Autodesk Inventor part; units mm, degrees
ref_plane "YZ Plane" through (0, 0, 0) normal (1, 0, 0) x (0, 1, 0)
ref_plane "XZ Plane" through (0, 0, 0) normal (0, 1, 0) x (-1, 0, 0)
ref_plane "XY Plane" through (0, 0, 0) normal (0, 0, 1) x (1, 0, 0)
sketch "Sketch1" plane through (0, 0, 0) normal (0, 0, 1) x (1, 0, 0)
  circle A0 centre (0, 0) radius 30
  dimension "d0" = 60
extrude "Extrusion1" add sketch "Sketch1" along normal mid plane 58.037
sketch "Sketch2" plane through (0, 0, 0) normal (0, 0, 1) x (1, 0, 0)
  circle A0 centre (0, 0) radius 30
  circle A1 centre (0, 0) radius 12
  dimension "d3" = 24
extrude "Extrusion2" add sketch "Sketch2" along normal mid plane 62.037 contours A1
sketch "Sketch3" plane through (0, 0, 0) normal (0, 0, 1) x (1, 0, 0)
  circle A0 centre (0, 0) radius 12
  circle A1 centre (0, 0) radius 9
  dimension "d6" = 18
extrude "Extrusion3" cut sketch "Sketch3" along normal mid plane 94.75 contours A1
sketch "Sketch4" plane through (0, 0, 0) normal (0, 0, 1) x (1, 0, 0)
  circle A0 centre (0, 0) radius 23.75
  circle A1 centre (0, 23.75) radius 2.5
  dimension "d9" = 47.5
  dimension "d10" = 5
extrude "Extrusion4" cut sketch "Sketch4" along normal mid plane 127.5 contours A1 A0 | A0 A1 picked at (-0.0971, 22.9126) picked at (0.0803, 24.5697)
pattern_circular "Circular Pattern1" count 12 over 360 about axis through (0, 0, 0) along (0, 0, 1) of "Extrusion4"
properties part number "shaft" material "Steel"
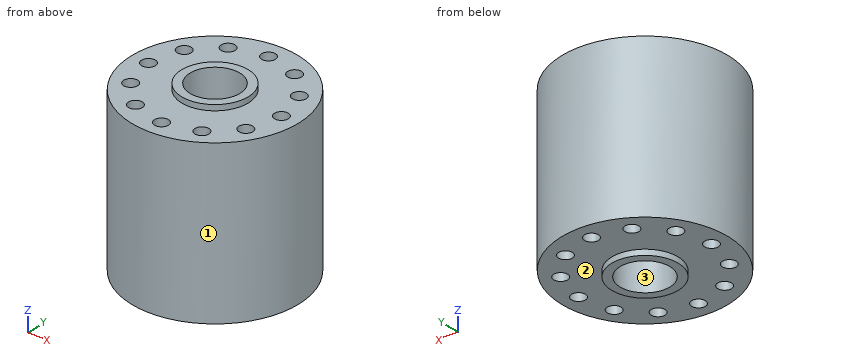
Geometry: final body of the model. Coordinates: model frame, mm. Face numbers are marked on the shaded views. Give positions to 0.01 mm unless a question says otherwise; leave off trailing zeros. Order: outer loops, then holes, each group sorted by start corner. A loop starts at its lowest first (then second) coordinate and runs counter-clockwise, first axis right, second up. Notation, with made-up numbers: M 71.25,80 L 90.25,80 A21 cw 90.25,109 Z; hole C 43,-28.75 d4. An arc over 180 degrees is marked long. Answer as CSV lines item,"result". Start each with the question number.
1) First-contact query: P1, Ø8, axis at x = 16, y = 6, coming from the -Z side; P2, Ø8, axis at x = 22.5, z = -18, coming from the -Y side; P3, Ø12, axis at y = 18.5, z = 7, coming from the +X side. Flat tips, straight axial feed; report the tip coordinate or a pass-through.
2) Cut plane C-C (z = -22.5). State how many separate pieces and enclosed holes the cut face has, then the cut area to 3 significant figures.
3) Line query: line 1 (Y direction, x = 1, z = -23); line 2 (X direction, y = -14, z = 8.5); line 3 (X direction, y = 12, z = -26.5). Output: solid intervals per line, ascending. Write a range as from..to.
4) Cut plane D-D (y = 16). Output: boundary loops of the cut face in (x, z).
5) Cut plane A-A (x = 0). Output: boundary loops of the cut face in (y, z).
6) Mould query, pull axis X, two halves, no side actions, for the marked faces 1, 2 and 3. Classes: +X half, -X half, draft (parallel to the pull), parting line (faces both ways), or undercut.
Findings below:
1,P1,"stops at z = -29.02"
1,P2,"stops at y = -23.62"
1,P3,"stops at x = 27.27"
2,separate pieces,"1"
2,enclosed holes,"13"
2,area,"2,340 mm²"
3,line 1,"y = -29.98..-26.04, -21.46..-8.94, 8.94..21.46, 26.04..29.98"
3,line 2,"x = -26.53..-21.89, -19.25..19.25, 21.89..26.53"
3,line 3,"x = -27.5..-23.06, -18.07..18.07, 23.06..27.5"
4,outline,"M -25.38,-29.02 L 25.38,-29.02 L 25.38,29.02 L -25.38,29.02 Z"
5,outline,"M -30,-29.02 L -26.25,-29.02 L -26.25,29.02 L -30,29.02 Z; M -21.25,-29.02 L -12,-29.02 L -12,-31.02 L -9,-31.02 L -9,31.02 L -12,31.02 L -12,29.02 L -21.25,29.02 Z; M 9,-31.02 L 12,-31.02 L 12,-29.02 L 21.25,-29.02 L 21.25,29.02 L 12,29.02 L 12,31.02 L 9,31.02 Z; M 26.25,-29.02 L 30,-29.02 L 30,29.02 L 26.25,29.02 Z"
6,face 1,"parting line"
6,face 2,"draft"
6,face 3,"undercut"
